```python
from build123d import *

# Parameters (mm, degrees)
F0_W      = 25.4
F0_H      = 50.8
F1_DEPTH  = 50.8
F2_R      = 6.35
F3_DEPTH  = 2.54
F4_R      = 6.35
F5_DEPTH  = 2.54
F6_R      = 6.35
F7_DEPTH  = 2.54
F8_R      = 6.35
F9_DEPTH  = 2.54
F10_R     = 6.35
F11_DEPTH = 2.54
F12_R     = 6.35
F13_DEPTH = 2.54


with BuildPart() as f1:
    # F0 (on Top) → F1 (new body)
    with BuildSketch(Plane.XY):
        with Locations((-12.7, 0)):
            Rectangle(F0_W, F0_H)
        with Locations((12.7, 0)):
            Rectangle(F0_W, F0_H)
    extrude(amount=F1_DEPTH)

    # F2 (on face) → F3 (cut)
    with BuildSketch(Plane.XY.offset(50.8)):
        Circle(F2_R)
    extrude(amount=-F3_DEPTH, mode=Mode.SUBTRACT)

    # F4 (on face) → F5 (cut)
    with BuildSketch(Plane(origin=(0, 0, 0), x_dir=(1, 0, 0), z_dir=(0, 0, -1))):
        with Locations((15.7828163356, 14.1213936731)):
            Circle(F4_R)
        with Locations((-14.078758657, 15.8332046121)):
            Circle(F4_R)
        with Locations((15.1571258903, 0)):
            Circle(F4_R)
        with Locations((-14.2689589411, 0)):
            Circle(F4_R)
        with Locations((-13.359840028, -15.3967663646)):
            Circle(F4_R)
        with Locations((14.4382100552, -15.1571286842)):
            Circle(F4_R)
    extrude(amount=-F5_DEPTH, mode=Mode.SUBTRACT)

    # F6 (on face) → F7 (cut)
    with BuildSketch(Plane.XZ.offset(25.4)):
        with Locations((18.1605778635, 6.8199974485)):
            Circle(F6_R)
        with Locations((-18.7246706337, 7.1070431732)):
            Circle(F6_R)
        with Locations((0, 22.4099811167)):
            Circle(F6_R)
        with Locations((16.5282599628, 44.2445091903)):
            Circle(F6_R)
        with Locations((-18.8880376518, 44.3454124033)):
            Circle(F6_R)
    extrude(amount=-F7_DEPTH, mode=Mode.SUBTRACT)

    # F8 (on face) → F9 (cut)
    with BuildSketch(Plane.YZ.offset(25.4)):
        with Locations((-16.7743396014, 40.8508107066)):
            Circle(F8_R)
        with Locations((14.7602735087, 40.6206287444)):
            Circle(F8_R)
        with Locations((-15.3932608664, 9.4312885776)):
            Circle(F8_R)
        with Locations((16.0262603313, 8.395479992)):
            Circle(F8_R)
    extrude(amount=-F9_DEPTH, mode=Mode.SUBTRACT)

    # F10 (on face) → F11 (cut)
    with BuildSketch(Plane(origin=(-25.4, 0, 0), x_dir=(0, -1, 0), z_dir=(-1, 0, 0))):
        with Locations((0, 25.7740411907)):
            Circle(F10_R)
        with Locations((16.2564348429, 10.3520061821)):
            Circle(F10_R)
        with Locations((-15.0479944423, 41.3111671805)):
            Circle(F10_R)
    extrude(amount=-F11_DEPTH, mode=Mode.SUBTRACT)

    # F12 (on face) → F13 (cut)
    with BuildSketch(Plane(origin=(0, 25.4, 0), x_dir=(-1, 0, 0), z_dir=(0, 1, 0))):
        with Locations((-17.407335341, 8.6256600916)):
            Circle(F12_R)
        with Locations((18.8459586352, 43.7280572951)):
            Circle(F12_R)
    extrude(amount=-F13_DEPTH, mode=Mode.SUBTRACT)


solid = f1.part
```
Input: part model. Units: mm. Frame: model coordinates. A direction names the side the tool comes from. Coordinates: 2 decimals unless noted, no trailing zeros. Loops run counter-clockwise (first coordinate to the right, second up) from the corner with the lowest first, then second, coordinate; pieces in that order, holes last.
Q1. Section C-C, the plane z = 28. Return the cut outline in (x, y).
Results are:
outline: (-25.4, -25.4) - (-3.01, -25.4) - (-3.01, -22.86) - (3.01, -22.86) - (3.01, -25.4) - (25.4, -25.4) - (25.4, 25.4) - (-25.4, 25.4) - (-25.4, 5.95) - (-22.86, 5.95) - (-22.86, -5.95) - (-25.4, -5.95) - close
Q2. Contact query for flat-ended pins moving along their axis: pin 1 (6 mm diameter, centred on x = 18, z = 6, fed in from +Y); pin 2 (10 mm diameter, centred on y = 16.5, z = 8.5, fed in from +X). Output: stop coordinate, or through.
Results are:
pin 1: stops at y = 22.86
pin 2: stops at x = 22.86
Q3. Set-up query: faces 1 (the flat face through (16, -14, 2.54)), 2 (the cylindrical face through (24.148, -9.527, 6.999)), 3 (the cylindrical face through (-21.776, 24.148, 38.095)). Return all of +Z, -Z, +X, -X, +Y, -Y with unobstructed straight access to the full face (end or side cutting, diameter ignored); none if empty.
Results are:
face 1: -Z
face 2: +X
face 3: +Y
Q4. Section A-A, the plane y = 0. Return the cut outline in (x, z).
Results are:
outline: (-25.4, 0) - (-20.62, 0) - (-20.62, 2.54) - (-7.92, 2.54) - (-7.92, 0) - (8.81, 0) - (8.81, 2.54) - (21.51, 2.54) - (21.51, 0) - (25.4, 0) - (25.4, 50.8) - (6.35, 50.8) - (6.35, 48.26) - (-6.35, 48.26) - (-6.35, 50.8) - (-25.4, 50.8) - (-25.4, 32.12) - (-22.86, 32.12) - (-22.86, 19.42) - (-25.4, 19.42) - close
Q5. Section B-B, the plane x = 4.5. Return the cut outline in (y, z), and give its area (3 significant figures).
Results are:
outline: (-25.4, 0) - (25.4, 0) - (25.4, 50.8) - (4.48, 50.8) - (4.48, 48.26) - (-4.48, 48.26) - (-4.48, 50.8) - (-25.4, 50.8) - (-25.4, 26.89) - (-22.86, 26.89) - (-22.86, 17.93) - (-25.4, 17.93) - close
area: 2,540 mm2
Q6. Mould query, pull axis Y, two halves, no side actions, for faces 4 (the flat face through (-14, 0, 2.54)), 5 (the cylindrical face through (-19.71, -24.15, 50.64)), 6 (the flat face through (16, -22.86, 44)). Classes: +Y half, -Y half, draft (parallel to the pull), parting line (faces both ways), or undercut.
Results are:
face 4: undercut
face 5: draft
face 6: -Y half
Q7. Line query: line 1 along Z through (x, y) = (-23, 0); line 2 along X through (y, z) = (14, 12); line 3 along X through (y, z) = (-14, 5.5). Output: solid intervals per line, ascending.
Results are:
line 1: z = 0 to 19.42, 32.12 to 50.8
line 2: x = -25.4 to 22.86
line 3: x = -22.86 to 22.86
Q8. Section D-D, the plane y = -18.5. Return the cut outline in (x, z), and give its area (3 significant figures).
Results are:
outline: (-25.4, 0) - (-19.84, 0) - (-19.84, 2.54) - (-8.32, 2.54) - (-8.32, 0) - (11.18, 0) - (11.18, 2.54) - (20.38, 2.54) - (20.38, 0) - (25.4, 0) - (25.4, 3.89) - (22.86, 3.89) - (22.86, 14.97) - (25.4, 14.97) - (25.4, 34.74) - (22.86, 34.74) - (22.86, 46.96) - (25.4, 46.96) - (25.4, 50.8) - (-25.4, 50.8) - (-25.4, 16.29) - (-22.86, 16.29) - (-22.86, 4.41) - (-25.4, 4.41) - close
area: 2,440 mm2
